The model under review builds one solid part; all positions refer to its coordinate system, in mm. A direction names the side the tool comes from. Give positions to 0.01 mm unless a question says otherwise; leave off trailing zeros. Loops run counter-clockwise (first coordinate to the right, second up) from the corner with the lowest first, then second, coordinate; pieces in that order, holes last. Notation, with made-up numbers: (74.5, 17.25) - (78.5, 17.25) arc R21 cw to (78.5, 34.25) - close; hole circle Ø6 at (80, 85). An arc over 180 degrees is marked (long way). Answer as a JSON object with one key per item and string values.
from build123d import *

# Parameters (mm, degrees)
F1_DEPTH = 31
F2_DEPTH = 25
F4_DEPTH = 137.1753371482
F5_R     = 12
F6_R     = 7
F7_DEPTH = 77.8189306876
F8_W     = 38
F8_H     = 50
F9_DEPTH = 60.001


# Not quite as in the source:
# - a feature of the source that left no trace in its solid (it failed there, or was rolled back) is left out


with BuildPart() as f1:
    # F0 (on Right) → F1 (new body, symmetric)
    with BuildSketch(Plane.YZ):
        Polygon((38, 2.3923048454), (38, 14), (-38, 14), (-38, 8), (-38, -8), (-38, -14), (38, -14), (38, -8), align=None)
    extrude(amount=F1_DEPTH, both=True)

    # F0 (on Right) → F2 (join, symmetric)
    with BuildSketch(Plane.YZ):
        Polygon((-38, -8), (-38, 8), (-57, 8), (-122.8179306876, -30), (-113.5803263806, -46), (-47.762395693, -8), align=None)
        Polygon((52, 2.3923048454), (38, 2.3923048454), (38, -8), (58, -8), (123.8179306876, 30), (117.8179306876, 40.3923048454), align=None)
    extrude(amount=F2_DEPTH, both=True)

    # F3 (on face) → F4 (cut, through all)
    with BuildSketch(Plane(origin=(0, -17.7141016151, 30.6817240079), x_dir=(1, 0, 0), z_dir=(0, -0.5, 0.8660254038))):
        with BuildLine():
            Line((10, -121.3634480157), (10, -76.3634480157))
            ThreePointArc((10, -76.3634480157), (0, -86.3634480157), (-10, -76.3634480157))
            Line((-10, -76.3634480157), (-10, -121.3634480157))
            Line((-10, -121.3634480157), (10, -121.3634480157))
        make_face()
        with BuildLine():
            ThreePointArc((-10, -76.3634480157), (0, -86.3634480157), (10, -76.3634480157))
            ThreePointArc((10, -76.3634480157), (0, -66.3634480157), (-10, -76.3634480157))
        make_face()
    extrude(amount=-F4_DEPTH, mode=Mode.SUBTRACT)

    # F5
    f5_edges = [f1.edges().sort_by_distance(p)[0] for p in [
        (25, -118.199129, -38),
        (-25, -118.199129, -38),
    ]]
    fillet(f5_edges, radius=F5_R)

    # F6 (on face) → F7 (cut, through all)
    with BuildSketch(Plane(origin=(0, 11.9641016151, -20.7224318643), x_dir=(1, 0, 0), z_dir=(0, -0.5, 0.8660254038))):
        with Locations((-13, 110.2294734195)):
            Circle(F6_R)
        with Locations((13, 110.2294734195)):
            Circle(F6_R)
        with Locations((13, 72.2294734195)):
            Circle(F6_R)
        with Locations((-13, 72.2294734195)):
            Circle(F6_R)
    extrude(amount=-F7_DEPTH, mode=Mode.SUBTRACT)

    # F8 (on face) → F9 (cut, through all)
    with BuildSketch(Plane.XY.offset(14)):
        Rectangle(F8_W, F8_H)
    extrude(amount=-F9_DEPTH, mode=Mode.SUBTRACT)


solid = f1.part
Q1. Consider section C-C, the plane x = 15.5. State the section outline as (y, z) points, plus the area to 3 significant figures.
Results:
{"outline": "(-122.59, -29.87) - (-113.35, -45.87) - (-47.76, -8) - (-38, -8) - (-38, -14) - (-25, -14) - (-25, 14) - (-38, 14) - (-38, 8) - (-57, 8) - close; (25, -14) - (38, -14) - (38, -8) - (58, -8) - (74.85, 1.73) - (68.85, 12.12) - (52, 2.39) - (38, 2.39) - (38, 14) - (25, 14) - close; (80.18, 18.66) - (86.18, 8.27) - (107.76, 20.73) - (101.76, 31.12) - close; (113.09, 37.66) - (119.09, 27.27) - (123.82, 30) - (117.82, 40.39) - close", "area": "3,130 mm^2"}
Q2. Consider section A-A, the plane y = 9. State the section outline as (x, z) points, plus the area to 3 significant figures.
Results:
{"outline": "(-31, -14) - (-19, -14) - (-19, 14) - (-31, 14) - close; (19, -14) - (31, -14) - (31, 14) - (19, 14) - close", "area": "672 mm^2"}
Q3. The part is to be moulded in two halves that separate along Z. For faces 5 (the face through (16.23, 105.01, 26.16)), 6 (the face through (11.48, 71.56, 6.85)), 7 (the face through (0.35, 85.37, 21.66)), 8 (the face through (0, 38, 3)), say which applies: +Z half, -Z half, draft (parallel to the pull), parting line (faces both ways), or undercut.
Results:
{"face 5": "undercut", "face 6": "undercut", "face 7": "+Z half", "face 8": "draft"}
Q4. Consider section B-B, the plane x = -3. State the section outline as (y, z) points, plus the area to 3 significant figures.
Results:
{"outline": "(-75.59, -2.73) - (-66.35, -18.73) - (-47.76, -8) - (-38, -8) - (-38, -14) - (-25, -14) - (-25, 14) - (-38, 14) - (-38, 8) - (-57, 8) - close; (25, -14) - (38, -14) - (38, -8) - (58, -8) - (123.82, 30) - (117.82, 40.39) - (52, 2.39) - (38, 2.39) - (38, 14) - (25, 14) - close", "area": "2,440 mm^2"}
Q5. Clearance check with flat-ended pins moving along their axes: pin 1 Ø3 at (x, y) = (-9, -87) entering from -Z; pin 2 Ø5 at (y, z) = (66, -1.5) entering from +X; pin 3 Ø4 at (x, y) = (4, 44) entering from +Z. State where each tip first meets the part, or that it passes through.
Results:
{"pin 1": "stops at z = -31.3", "pin 2": "stops at x = 25", "pin 3": "stops at z = 2.39"}
Q6. To check wall thickness, follow probe 1 along Y at (x, z) = (-7.5, -11.5); probe 2 along Y at (x, z) = (8.5, 11); probe 3 along X at (y, z) = (97, 15). State the ranges of each line that lie inside material, in increasing order. Write a range as [from, to].
Results:
{"probe 1": "y = [-73.9, -53.82], [-38, -25], [25, 38]", "probe 2": "y = [-38, -25], [25, 38], [66.91, 70.86], [83.24, 90.91]", "probe 3": "x = [-25, 25]"}
Q7. Consider section D-D, the plane y = -93.5. State the section outline as (x, z) points, plus the area to 3 significant figures.
Results:
{"outline": "(-25, -34.41) - (-10, -34.41) - (-10, -13.07) - (-25, -13.07) - close; (10, -34.41) - (25, -34.41) - (25, -13.07) - (10, -13.07) - close", "area": "640 mm^2"}
Q8. For faces 1 (the face through (-11.461, -73.819, -23.044)), 2 (the face through (-25, -76, -10)), 3 (the face through (25, -76, -10)), 4 (the face through (19, 0, 0)), list the 3-axis set-ups (+Z, -Z, +X, -X, +Y, -Y) from which the entire face can be reached by the end or side of a thin tool; tool diameter is ignored.
Results:
{"face 1": "-Z, +X, -X", "face 2": "+Z, -Z, -X, -Y", "face 3": "+Z, -Z, +X, -Y", "face 4": "+Z, -Z"}
